```python
from build123d import *

# Parameters (mm, degrees)
F0_W     = 350
F0_H     = 80
F1_DEPTH = 80


with BuildPart() as f1:
    # F0 (on Top) → F1 (new body)
    with BuildSketch(Plane.XY):
        Polygon((0, 650), (0, 0), (80, 0), (80, 269.4520485401), (79.9472002188, 269.4520485401), (80, 349.4520485401), (80, 470), (80, 550), (80, 650), align=None)
        Polygon((79.9472002188, 269.4520485401), (80, 269.4520485401), (80, 349.4520485401), align=None)
        with Locations((255, 309.4520485401)):
            Rectangle(F0_W, F0_H)
        Polygon((430, 349.4520485401), (430, 269.4520485401), (430, 0), (510, 0), (510, 650), (430, 650), (430, 550), (430, 470), align=None)
        with Locations((255, 510)):
            Rectangle(F0_W, F0_H)
    extrude(amount=F1_DEPTH)


solid = f1.part
```
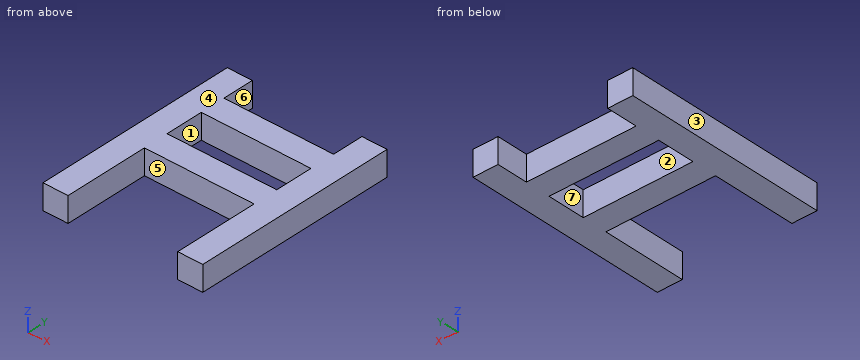
Here's how the part is built. I have some questions about the finished solid (model axes, mm). Face numbers are marked on the shaded views. A direction names the side the tool comes from. Coordinates: 2 decimals unless noted, no trailing zeros. Write each loop counter-clockwise with the first axis right and the second up, starting at its lowest first coordinate (ties: lowest second). Pieces come first, ordered by that corner, then holes. Notation, with made-up numbers: M 4,4 L 35,4 A17 cw 35,35 Z; hole C 17.25,20 d10. An arc over 180 degrees is marked long. Answer as CSV lines item,"result". Start each with the question number.
Q1. Will these pins go through, and if not, where does the flat tip stop? pin 1 Ø1.5 at (x, z) = (245.5, 51.5) entering from -Y; pin 2 Ø12 at (x, z) = (326, 24.5) entering from +Y.
Q2. Suppose I cut it at C-C, the plane z = 48.5. List the corners of the cut face in (x, y) for me, then the cut area to 3 significant figures.
Q3. Suppose I cut it at A-A, the plane y = 457.5. List the corners of the cut face in (x, z) for me.
Q4. If we mould it in two halves opening along X, with no side actions, what happens to the marked faces 1, 2, 3 and 4? For each: pulls with the +X half, pulls with the -X half, needs draft (parallel to the pull), parting line crosses it, or undercut.
Q5. For the marked faces 5, 6 and 7, which set-ups out of +Z, -Z, +X, -X, +Y, -Y let a thin tool reach every point of the face, with its end or its side?
Q6. Suppose I cut it at B-B, the plane x = 177.5. List the corners of the cut face in (y, z) for me.
Q7. I need wall thicknesses on probe 1 along X at (y, z) = (143, 69); probe 2 along Y at (x, z) = (114, 27.5). Which ranges of each line are inside material? Lowest first, please. Write a range as [from, to].
Entries:
1,pin 1,"stops at y = 269.45"
1,pin 2,"stops at y = 550"
2,outline,"M 0,0 L 80,0 L 80,269.45 L 430,269.45 L 430,0 L 510,0 L 510,650 L 430,650 L 430,550 L 80,550 L 80,650 L 0,650 Z; hole M 80,349.45 L 430,349.45 L 430,470 L 80,470 Z"
2,area,"160,000 mm²"
3,outline,"M 0,0 L 80,0 L 80,80 L 0,80 Z; M 430,0 L 510,0 L 510,80 L 430,80 Z"
4,face 1,"undercut"
4,face 2,"undercut"
4,face 3,"pulls with the -X half"
4,face 4,"needs draft"
5,face 5,"+Z, -Z, -Y"
5,face 6,"+Z, -Z, +Y"
5,face 7,"+Z, -Z"
6,outline,"M 269.45,0 L 349.45,0 L 349.45,80 L 269.45,80 Z; M 470,0 L 550,0 L 550,80 L 470,80 Z"
7,probe 1,"x = [0, 80], [430, 510]"
7,probe 2,"y = [269.45, 349.45], [470, 550]"
